Geometry: final body of the model. Coordinates: model frame, mm. A direction names the side the tool comes from. Round coordinates to 2 decimals unless told otherwise and drop trailing zeros. Loops run counter-clockwise (first coordinate to the right, second up) from the corner with the lowest first, then second, coordinate; pieces in that order, holes last. Notation, with made-up numbers: (80, 4.5) - (93, 4.5) arc R22 cw to (93, 18.5) - close; hole circle Ø7 at (12.25, 55.5). An arc over 180 degrees is marked (long way). Answer as a JSON object with one key per item and string values. Group by question number.
Item 1: Reachability of faces 4 (the face through (9.9, 5.5, -8)), 5 (the face through (15.8, -2, -13)), 6 (the face through (3.45, 3, -13)), 7 (the face through (9, 0, -4)) from +Z, -Z, +X, -X, +Y, -Y: full face, straight path, thin tool, end or side. Return the list, or none.
Item 2: Draft query along Z for faces 1 (the face through (17.43, 1.52, -0.6)), 2 (the face through (10, 6, -9)), 3 (the face through (3.164, 1.479, -1.487)). Return one class per face: released by +Z, released by -Z, zero draft, split by the parting line, or undercut.
Item 3: Section C-C (x = 14.5). Return the cut outline in (y, z).
Item 4: Section A-A (x = 8.5). Return the cut outline in (y, z).
Item 5: Section D-D (y = -2). Return the cut outline in (x, z).
Item 6: First-contact query: pin 1 (1 mm diameter, centred on y = 5, z = -12.5, fed in from -X); pin 2 (0.5 mm diameter, centred on x = 8.5, y = 5.5, fed in from +Z); pin 3 (2 mm diameter, centred on x = 4.5, z = -10.5, fed in from -Y); pin 4 (3.5 mm diameter, centred on x = 3.5, z = -3, fed in from -Y). Flat tips, straight axial feed; report the tip coordinate or a pass-through.
Item 7: Section B-B (z = -3). Return the cut outline in (x, y), plus the area to 3 significant figures.
Item 8: Line query: line 1 (X direction, y = 2.1, z = -3); line 2 (Z direction, x = 9, y = -0.75); line 3 (X direction, y = 4, z = -11.5). Output: solid intervals per line, ascending.
```python
from build123d import *

# Parameters (mm, degrees)
CROQUIS1_W              = 18
CROQUIS1_H              = 18
CROQUIS1_R              = 1.55
SALIENTE_EXTRUIR1_DEPTH = 3
CROQUIS3_W              = 18
CROQUIS3_H              = 10
SALIENTE_EXTRUIR3_DEPTH = 3
CROQUIS4_W              = 2
CROQUIS4_H              = 10
CORTAR_EXTRUIR1_DEPTH   = 6
CROQUIS7_W              = 13.1
CROQUIS7_H              = 6.1
CORTAR_EXTRUIR2_DEPTH   = 6
CROQUIS9_W              = 16
CROQUIS9_H              = 10
CROQUIS9_W_2            = 13.1
CROQUIS9_H_2            = 6.1
SALIENTE_EXTRUIR4_DEPTH = 3
CROQUIS10_W             = 13.1
CROQUIS10_H             = 6.1
CROQUIS10_W_2           = 11.6
CROQUIS10_H_2           = 4.6
SALIENTE_EXTRUIR6_DEPTH = 2.5
CROQUIS11_W             = 16
CROQUIS11_H             = 1
CORTAR_EXTRUIR4_DEPTH   = 9
REDONDEO1_R             = 2
CROQUIS12_W             = 8
CROQUIS12_H             = 3
CORTAR_EXTRUIR5_DEPTH   = 1
REDONDEO2_R             = 2


with BuildPart() as part:
    # Croquis1 → Saliente-Extruir1 (new body)
    with BuildSketch(Plane(origin=(0, 0, 0), x_dir=(1, 0, 0), z_dir=(0, 1, 0))):
        with Locations((9, 9)):
            Rectangle(CROQUIS1_W, CROQUIS1_H)
        with Locations((3.5, 3)):
            Circle(CROQUIS1_R, mode=Mode.SUBTRACT)
        with Locations((14.5, 3)):
            Circle(CROQUIS1_R, mode=Mode.SUBTRACT)
    extrude(amount=SALIENTE_EXTRUIR1_DEPTH)

    # Croquis3 → Saliente-Extruir3 (add)
    with BuildSketch(Plane(origin=(0, 3, 0), x_dir=(1, 0, 0), z_dir=(0, 1, 0))):
        with Locations((9, 13)):
            Rectangle(CROQUIS3_W, CROQUIS3_H)
    extrude(amount=SALIENTE_EXTRUIR3_DEPTH)

    # Croquis4 → Cortar-Extruir1 (cut)
    with BuildSketch(Plane.XZ):
        with Locations((1, -13)):
            Rectangle(CROQUIS4_W, CROQUIS4_H)
    extrude(amount=-CORTAR_EXTRUIR1_DEPTH, mode=Mode.SUBTRACT)

    # Croquis7 → Cortar-Extruir2 (cut)
    with BuildSketch(Plane(origin=(0, 6, 0), x_dir=(1, 0, 0), z_dir=(0, 1, 0))):
        with Locations((10, 12.55)):
            Rectangle(CROQUIS7_W, CROQUIS7_H)
    extrude(amount=-CORTAR_EXTRUIR2_DEPTH, mode=Mode.SUBTRACT)

    # Croquis9 → Saliente-Extruir4 (add)
    with BuildSketch(Plane.XZ):
        with Locations((10, -13)):
            Rectangle(CROQUIS9_W, CROQUIS9_H)
        with Locations((10, -12.55)):
            Rectangle(CROQUIS9_W_2, CROQUIS9_H_2, mode=Mode.SUBTRACT)
    extrude(amount=SALIENTE_EXTRUIR4_DEPTH)

    # Croquis10 → Saliente-Extruir6 (add)
    with BuildSketch(Plane.XZ.offset(3)):
        with Locations((10, -12.55)):
            Rectangle(CROQUIS10_W, CROQUIS10_H)
        with Locations((10, -12.55)):
            Rectangle(CROQUIS10_W_2, CROQUIS10_H_2, mode=Mode.SUBTRACT)
    extrude(amount=-SALIENTE_EXTRUIR6_DEPTH)

    # Croquis11 → Cortar-Extruir4 (cut)
    with BuildSketch(Plane(origin=(0, 6, 0), x_dir=(1, 0, 0), z_dir=(0, 1, 0))):
        with Locations((10, 17.5)):
            Rectangle(CROQUIS11_W, CROQUIS11_H)
    extrude(amount=-CORTAR_EXTRUIR4_DEPTH, mode=Mode.SUBTRACT)

    # Redondeo1
    redondeo1_edges = [part.edges().sort_by_distance(p)[0] for p in [
        (18, 1.5, -17),
        (2, 1.5, -17),
        (18, 1.5, 0),
    ]]
    fillet(redondeo1_edges, radius=REDONDEO1_R)

    # Croquis12 → Cortar-Extruir5 (cut)
    with BuildSketch(Plane.ZY):
        with Locations((-4, 1.5)):
            Rectangle(CROQUIS12_W, CROQUIS12_H)
    extrude(amount=-CORTAR_EXTRUIR5_DEPTH, mode=Mode.SUBTRACT)

    # Redondeo2
    redondeo2_edges = [part.edges().sort_by_distance(p)[0] for p in [
        (10, 3, -8),
    ]]
    fillet(redondeo2_edges, radius=REDONDEO2_R)


solid = part.part
```
Values:
{
 "1": {"face 4": "+Z, +X, -X, +Y", "face 5": "+Y, -Y", "face 6": "+Y", "face 7": "+Z, +X, -X, -Y"},
 "2": {"face 1": "released by +Z", "face 2": "zero draft", "face 3": "undercut"},
 "3": {"outline": "(-3, -17) - (6, -17) - (6, -15.6) - (-0.5, -15.6) - (-0.5, -14.85) - (-3, -14.85) - close; (-3, -10.25) - (-0.5, -10.25) - (-0.5, -9.5) - (6, -9.5) - (6, -8) - (5, -8) arc R2 cw to (3, -6) - (3, -4.55) - (0, -4.55) - (0, -8) - (-3, -8) - close; (0, -1.45) - (3, -1.45) - (3, 0) - (0, 0) - close"},
 "4": {"outline": "(-3, -17) - (6, -17) - (6, -15.6) - (-0.5, -15.6) - (-0.5, -14.85) - (-3, -14.85) - close; (-3, -10.25) - (-0.5, -10.25) - (-0.5, -9.5) - (6, -9.5) - (6, -8) - (5, -8) arc R2 cw to (3, -6) - (3, 0) - (0, 0) - (0, -8) - (-3, -8) - close"},
 "5": {"outline": "(2, -15) arc R2 ccw to (4, -17) - (16, -17) arc R2 ccw to (18, -15) - (18, -8) - (2, -8) - close; hole (4.2, -14.85) - (15.8, -14.85) - (15.8, -10.25) - (4.2, -10.25) - close"},
 "6": {"pin 1": "stops at x = 2", "pin 2": "stops at z = -8", "pin 3": "stops at y = -3", "pin 4": "stops at y = 0"},
 "7": {"outline": "(1, 0) - (1.95, 0) - (1.95, 3) - (1, 3) - close; (5.05, 0) - (12.95, 0) - (12.95, 3) - (5.05, 3) - close; (16.05, 0) - (18, 0) - (18, 3) - (16.05, 3) - close", "area": "32.4 mm^2"},
 "8": {"line 1": "x = 1 to 1.95, 5.05 to 12.95, 16.05 to 18", "line 2": "z = -17 to -14.85, -10.25 to -8", "line 3": "x = 2 to 3.45, 16.55 to 18"}
}
